```python
from build123d import *

# Parameters (mm, degrees)
CROQUIS1_R              = 2.5
SALIENTE_EXTRUIR2_DEPTH = 10
CROQUIS3_W              = 104.7
CROQUIS3_H              = 8
SALIENTE_EXTRUIR3_DEPTH = 45
CROQUIS4_W              = 104.7
CROQUIS4_H              = 7
SALIENTE_EXTRUIR4_DEPTH = 40
CROQUIS6_R              = 20
CORTAR_EXTRUIR1_DEPTH   = 92.797287028
REDONDEO2_R             = 3
CORTAR_EXTRUIR3_DEPTH   = 100.186815901
CROQUIS12_W             = 67.999748742
CROQUIS12_H             = 7
CORTAR_EXTRUIR4_DEPTH   = 104.841342675
REDONDEO5_R             = 5
CROQUIS13_W             = 67.999748742
CROQUIS13_H             = 8
CORTAR_EXTRUIR6_DEPTH   = 7
CROQUIS18_W             = 67.999748742
CROQUIS18_H             = 8
SALIENTE_EXTRUIR7_DEPTH = 45
CORTAR_EXTRUIR7_REACH   = 122.557
CROQUIS19_R             = 1.25
CROQUIS19_R_2           = 6.5
REDONDEO8_R             = 5
REDONDEO10_R            = 3


with BuildPart() as part:
    # Croquis1 → Saliente-Extruir2 (new body)
    with BuildSketch(Plane.XY):
        Polygon((74.222802753, 23.027181924), (49.222802753, 23.027181924), (49.222802753, -6.972818076), (-10.477197247, -6.972818076), (-10.477197247, 23.027181924), (-30.477197247, 23.027181924), (-30.477197247, -41.972818076), (74.222802753, -41.972818076), align=None)
        with Locations((-14.377197247, 16.777181924)):
            Circle(CROQUIS1_R, mode=Mode.SUBTRACT)
        with Locations((-14.377197247, -0.722818076)):
            Circle(CROQUIS1_R, mode=Mode.SUBTRACT)
        with Locations((53.122802753, 16.777181924)):
            Circle(CROQUIS1_R, mode=Mode.SUBTRACT)
        with Locations((53.122802753, -0.722818076)):
            Circle(CROQUIS1_R, mode=Mode.SUBTRACT)
    extrude(amount=SALIENTE_EXTRUIR2_DEPTH)

    # Croquis3 → Saliente-Extruir3 (add)
    with BuildSketch(Plane(origin=(0, 0, 0), x_dir=(-1, 0, 0), z_dir=(0, 0, -1))):
        with Locations((-21.872802753, -37.972818076)):
            Rectangle(CROQUIS3_W, CROQUIS3_H)
    extrude(amount=SALIENTE_EXTRUIR3_DEPTH)

    # Croquis4 → Saliente-Extruir4 (add)
    with BuildSketch(Plane(origin=(0, -33.972818076, 0), x_dir=(1, 0, 0), z_dir=(0, 1, 0))):
        with Locations((21.872802753, 27.5)):
            Rectangle(CROQUIS4_W, CROQUIS4_H)
    extrude(amount=SALIENTE_EXTRUIR4_DEPTH)

    # Croquis6 → Cortar-Extruir1 (cut, through all)
    with BuildSketch(Plane.XY.offset(-24)):
        with Locations((3.522802753, 8.027181924)):
            Circle(CROQUIS6_R)
    extrude(amount=-CORTAR_EXTRUIR1_DEPTH, mode=Mode.SUBTRACT)

    # Redondeo2
    redondeo2_edges = [part.edges().sort_by_distance(p)[0] for p in [
        (74.222802753, 23.027181924, 5),
        (-30.477197247, 23.027181924, 5),
    ]]
    fillet(redondeo2_edges, radius=REDONDEO2_R)

    # Croquis10 → Cortar-Extruir3 (cut, through all)
    with BuildSketch(Plane(origin=(0, 6.027181924, 0), x_dir=(1, 0, 0), z_dir=(0, 1, 0))):
        Polygon((74.222802753, 45), (37.522551495, 45), (37.522551495, 15.052232973), (74.222802753, 0), align=None)
    extrude(amount=-CORTAR_EXTRUIR3_DEPTH, mode=Mode.SUBTRACT)

    # Croquis12 → Cortar-Extruir4 (cut, through all)
    with BuildSketch(Plane(origin=(0, -33.972818076, 0), x_dir=(1, 0, 0), z_dir=(0, 1, 0))):
        with Locations((3.522677124, 41.5)):
            Rectangle(CROQUIS12_W, CROQUIS12_H)
    extrude(amount=-CORTAR_EXTRUIR4_DEPTH, mode=Mode.SUBTRACT)

    # Redondeo5
    redondeo5_edges = [part.edges().sort_by_distance(p)[0] for p in [
        (37.522551495, -37.972818076, -15.052232973),
    ]]
    fillet(redondeo5_edges, radius=REDONDEO5_R)

    # Croquis13 → Cortar-Extruir6 (cut)
    with BuildSketch(Plane(origin=(0, 0, -38), x_dir=(-1, 0, 0), z_dir=(0, 0, -1))):
        with Locations((-3.522677124, -37.972818076)):
            Rectangle(CROQUIS13_W, CROQUIS13_H)
    extrude(amount=-CORTAR_EXTRUIR6_DEPTH, mode=Mode.SUBTRACT)

    # Croquis18 → Saliente-Extruir7 (add)
    with BuildSketch(Plane(origin=(0, 0, -31), x_dir=(-1, 0, 0), z_dir=(0, 0, -1))):
        with Locations((-3.522677124, -37.972818076)):
            Rectangle(CROQUIS18_W, CROQUIS18_H)
    extrude(amount=SALIENTE_EXTRUIR7_DEPTH)

    # Croquis19 → Cortar-Extruir7 (cut, up to next)
    with BuildSketch(Plane(origin=(0, -33.972818076, 0), x_dir=(1, 0, 0), z_dir=(0, 1, 0)), mode=Mode.PRIVATE) as cortar_extruir7_sk1:
        with Locations(Location((-25.977197247, 54, 0), (0, 0, 270))):
            Circle(CROQUIS19_R)
    cortar_extruir7_tool1 = extrude(cortar_extruir7_sk1.sketch, amount=-CORTAR_EXTRUIR7_REACH, mode=Mode.PRIVATE) & part.part
    # Croquis19 → Cortar-Extruir7 (cut, up to next)
    with BuildSketch(Plane(origin=(0, -33.972818076, 0), x_dir=(1, 0, 0), z_dir=(0, 1, 0)), mode=Mode.PRIVATE) as cortar_extruir7_sk2:
        with Locations((33.022802753, 54)):
            Circle(CROQUIS19_R)
    cortar_extruir7_tool2 = extrude(cortar_extruir7_sk2.sketch, amount=-CORTAR_EXTRUIR7_REACH, mode=Mode.PRIVATE) & part.part
    # Croquis19 → Cortar-Extruir7 (cut, up to next)
    with BuildSketch(Plane(origin=(0, -33.972818076, 0), x_dir=(1, 0, 0), z_dir=(0, 1, 0)), mode=Mode.PRIVATE) as cortar_extruir7_sk3:
        with Locations(Location((-20.977197247, 54, 0), (0, 0, 270))):
            Circle(CROQUIS19_R)
    cortar_extruir7_tool3 = extrude(cortar_extruir7_sk3.sketch, amount=-CORTAR_EXTRUIR7_REACH, mode=Mode.PRIVATE) & part.part
    # Croquis19 → Cortar-Extruir7 (cut, up to next)
    with BuildSketch(Plane(origin=(0, -33.972818076, 0), x_dir=(1, 0, 0), z_dir=(0, 1, 0)), mode=Mode.PRIVATE) as cortar_extruir7_sk4:
        with Locations((28.022802753, 54)):
            Circle(CROQUIS19_R)
    cortar_extruir7_tool4 = extrude(cortar_extruir7_sk4.sketch, amount=-CORTAR_EXTRUIR7_REACH, mode=Mode.PRIVATE) & part.part
    # Croquis19 → Cortar-Extruir7 (cut, up to next)
    with BuildSketch(Plane(origin=(0, -33.972818076, 0), x_dir=(1, 0, 0), z_dir=(0, 1, 0)), mode=Mode.PRIVATE) as cortar_extruir7_sk5:
        with Locations(Location((3.522802753, 54, 0), (0, 0, 270))):
            Circle(CROQUIS19_R_2)
    cortar_extruir7_tool5 = extrude(cortar_extruir7_sk5.sketch, amount=-CORTAR_EXTRUIR7_REACH, mode=Mode.PRIVATE) & part.part
    add(cortar_extruir7_tool1.solids().sort_by_distance((-25.977197, -33.972818, -54))[0], mode=Mode.SUBTRACT)
    add(cortar_extruir7_tool2.solids().sort_by_distance((33.022803, -33.972818, -54))[0], mode=Mode.SUBTRACT)
    add(cortar_extruir7_tool3.solids().sort_by_distance((-20.977197, -33.972818, -54))[0], mode=Mode.SUBTRACT)
    add(cortar_extruir7_tool4.solids().sort_by_distance((28.022803, -33.972818, -54))[0], mode=Mode.SUBTRACT)
    add(cortar_extruir7_tool5.solids().sort_by_distance((3.522803, -33.972818, -54))[0], mode=Mode.SUBTRACT)

    # Redondeo8
    redondeo8_edges = [part.edges().sort_by_distance(p)[0] for p in [
        (37.522551495, -37.972818076, -76),
        (-30.477197247, -37.972818076, -76),
    ]]
    fillet(redondeo8_edges, radius=REDONDEO8_R)

    # Redondeo10
    redondeo10_edges = [part.edges().sort_by_distance(p)[0] for p in [
        (-30.477197247, 6.027181924, -27.5),
        (37.522551495, 6.027181924, -27.5),
    ]]
    fillet(redondeo10_edges, radius=REDONDEO10_R)


solid = part.part
```
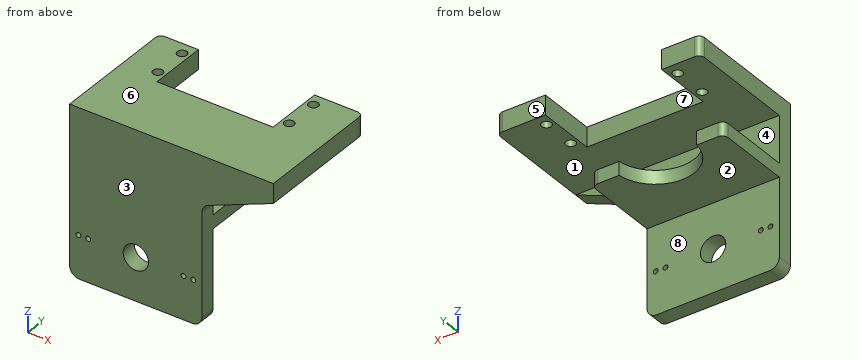
Geometry: final body of the model. Coordinates: model frame, mm. Face numbers are marked on the shaded views. A direction names the side the tool comes from. Round coordinates to 2 decimals unless told otherwise and drop trailing zeros. Write each loop counter-clockwise with the first axis right and the second up, starting at its lowest first coordinate (ties: lowest second). Pieces come first, ordered by that corner, then holes. Notation, with made-up numbers: M 30,33 L 42,33 A11 ccw 42,46 Z; hole C 54,20.5 d9. An arc over 180 degrees is marked long. Answer in a Markdown table with one row per item. Add a question column.
(1) Contact query for flat-ended pins moving along their axis: pin 1 (4.5 mm diameter, centred on x = -14.38, y = 16.78, fed in from +Z); pin 2 (3 mm diameter, centred on x = -14.38, y = -0.72, fed in from +Z); pin 3 (5.5 mm diameter, centred on x = -20, z = -27, fed in from +Y); pin 4 (2 mm diameter, centred on x = -16, z = -58.5, fed in from +Y). Output: stop coordinate, or through.
(2) Cut plane C-C, the plane x = -6. Return the cut outline in (y, z).
(3) Cut plane D-D, the plane z = -68. Return the cut outline in (x, y).
(4) Cut plane B-B, the plane z = -54. Return the cut outline in (x, y), then the cut area to 3 significant figures.
(5) Cut plane A-A, the plane y = -27.5. Return the cut outline in (x, z).
(6) Draft query along Z for the marked faces 1, 2 and 3. Return one class per face: pulls with the +Z half, pulls with the -Z half, needs draft (parallel to the pull), parting line crosses it, or undercut.
(7) Ray query, L1, parallel to X at y = -39.25, z = -54; L2, parallel to Z at x = -16.5, y = 1; L3, parallel to X at y = -3, z = 3.5. Return the intervals inside material, ascending.
(8) Reachability of the marked faces 4, 5, 6, 7 and 8 from +Z, -Z, +X, -X, +Y, -Y: full face, straight path, thin tool, end or side. Return the list, or none.
Established:
| question | item | result |
|---|---|---|
| 1 | pin 1 | through |
| 1 | pin 2 | z = -24 |
| 1 | pin 3 | y = 6.03 |
| 1 | pin 4 | y = -33.97 |
| 2 | outline | M -41.97,-76 L -33.97,-76 L -33.97,-31 L -9.56,-31 L -9.56,-24 L -33.97,-24 L -33.97,0 L -6.97,0 L -6.97,10 L -41.97,10 Z |
| 3 | outline | M -30.48,-41.97 L 37.52,-41.97 L 37.52,-33.97 L -30.48,-33.97 Z |
| 4 | outline | M -30.48,-41.97 L -27.23,-41.97 L -27.23,-33.97 L -30.48,-33.97 Z; M -24.73,-41.97 L -22.23,-41.97 L -22.23,-33.97 L -24.73,-33.97 Z; M -19.73,-41.97 L -2.98,-41.97 L -2.98,-33.97 L -19.73,-33.97 Z; M 10.02,-41.97 L 26.77,-41.97 L 26.77,-33.97 L 10.02,-33.97 Z; M 29.27,-41.97 L 31.77,-41.97 L 31.77,-33.97 L 29.27,-33.97 Z; M 34.27,-41.97 L 37.52,-41.97 L 37.52,-33.97 L 34.27,-33.97 Z |
| 4 | area | 360 mm² |
| 5 | outline | M -30.48,-31 L 37.52,-31 L 37.52,-24 L -30.48,-24 Z; M -30.48,0 L 74.22,0 L 74.22,10 L -30.48,10 Z |
| 6 | face 1 | undercut |
| 6 | face 2 | pulls with the -Z half |
| 6 | face 3 | needs draft |
| 7 | L1 | -30.48 to -27.23, -24.73 to -22.23, -19.73 to -2.98, 10.02 to 26.77, 29.27 to 31.77, 34.27 to 37.52 |
| 7 | L2 | -31 to -24, 0 to 10 |
| 7 | L3 | -30.48 to -15.41, -13.35 to -10.48, 49.22 to 52.09, 54.15 to 74.22 |
| 8 | face 4 | +X, -X, +Y |
| 8 | face 5 | +Z, -Z, +X, -X, +Y |
| 8 | face 6 | +Z, +X, -X, +Y, -Y |
| 8 | face 7 | +Z, +Y |
| 8 | face 8 | -Z, +X, -X, +Y |
